Here's how the part is built. I have some questions about the finished solid (model axes, mm). A direction names the side the tool comes from. Coordinates: 2 decimals unless noted, no trailing zeros. Loops run counter-clockwise (first coordinate to the right, second up) from the corner with the lowest first, then second, coordinate; pieces in that order, holes last.
from build123d import *

# Parameters (mm, degrees)
F0_W     = 457.2
F0_H     = 342.9
F1_DEPTH = 12.7
F2_W     = 355.6
F2_H     = 241.3
F3_DEPTH = 25.4
F4_W     = 25.4
F4_H     = 127
F5_DEPTH = 25.4
F6_R     = 12.7


with BuildPart() as f1:
    # F0 (on Top) → F1 (new body)
    with BuildSketch(Plane.XY):
        with Locations((184.6840278864, 135.7329336226)):
            Rectangle(F0_W, F0_H)
    extrude(amount=F1_DEPTH)

    # F2 (on face) → F3 (cut)
    with BuildSketch(Plane.XY.offset(12.7)):
        with Locations((184.6840278864, 135.7329336226)):
            Rectangle(F2_W, F2_H)
    extrude(amount=-F3_DEPTH, mode=Mode.SUBTRACT)

    # F4 (on face) → F5 (cut)
    with BuildSketch(Plane.XY.offset(12.7)):
        with Locations((-5.8159721136, 135.7329336226)):
            Rectangle(F4_W, F4_H)
        with Locations((375.1840278864, 135.7329336226)):
            Rectangle(F4_W, F4_H)
    extrude(amount=-F5_DEPTH, mode=Mode.SUBTRACT)

    # F6
    f6_edges = [f1.edges().sort_by_distance(p)[0] for p in [
        (-18.515972, 199.232934, 6.35),
        (387.884028, 199.232934, 6.35),
        (-18.515972, 72.232934, 6.35),
        (387.884028, 72.232934, 6.35),
    ]]
    fillet(f6_edges, radius=F6_R)


solid = f1.part
Q1. Please list where these lines run through material, in increasing order: probe 1 along Y at (x, z) = (128, 1.5); probe 2 along X at (y, z) = (182, 9.25); probe 3 along Y at (x, z) = (-3.5, 7.75).
Q2. We'd pull the mould along X, two halves only. Please class faces 3 (the flat face through (181, -35.717, 6)), 4 (the flat face through (-43.916, 133, 6)), 5 (the flat face through (362.484, 43, 6)): pulls with the +X half, pulls with the -X half, needs draft (parallel to the pull), parting line crosses it, or undercut.
Q3. Will this pin go through, and if not, where does the flat tip stop? P1, Ø8, axis at x = 180.5, y = 251, coming from the -Z side.
Q4. Suppose I cut it at C-C on z = 2. Write out the boundary of the cut face in (x, y), and give its area (3 significant figures).
Q5. Suppose I cut it at B-B on x = 29. Write out the boundary of the cut face in (y, z), and give its area (3 significant figures).
Q6. For faces 1 (the flat face through (184, 264, 12.7)), 2 (the flat face through (362.484, 227, 6)), which set-ups out of +Z, -Z, +X, -X, +Y, -Y let a thin tool reach every point of the face, with its end or its side?
Q7. Suppose I cut it at A-A on y = 32. Write out the boundary of the cut face in (x, z), and give its area (3 significant figures).
Check values:
1. probe 1: y = -35.72 to 15.08, 256.38 to 307.18
1. probe 2: x = -43.92 to -18.52, 387.88 to 413.28
1. probe 3: y = -35.72 to 72.23, 199.23 to 307.18
2. face 3: needs draft
2. face 4: pulls with the -X half
2. face 5: undercut
3. P1: passes through
4. outline: (-43.92, -35.72) - (413.28, -35.72) - (413.28, 307.18) - (-43.92, 307.18) - close; hole (-18.52, 84.93) arc R12.7 ccw to (-5.82, 72.23) - (6.88, 72.23) - (6.88, 15.08) - (362.48, 15.08) - (362.48, 72.23) - (375.18, 72.23) arc R12.7 ccw to (387.88, 84.93) - (387.88, 186.53) arc R12.7 ccw to (375.18, 199.23) - (362.48, 199.23) - (362.48, 256.38) - (6.88, 256.38) - (6.88, 199.23) - (-5.82, 199.23) arc R12.7 ccw to (-18.52, 186.53) - close
4. area: 64,700 mm2
5. outline: (-35.72, 0) - (15.08, 0) - (15.08, 12.7) - (-35.72, 12.7) - close; (256.38, 0) - (307.18, 0) - (307.18, 12.7) - (256.38, 12.7) - close
5. area: 1,290 mm2
6. face 1: +Z, +X, -X, +Y, -Y
6. face 2: +Z, -Z
7. outline: (-43.92, 0) - (6.88, 0) - (6.88, 12.7) - (-43.92, 12.7) - close; (362.48, 0) - (413.28, 0) - (413.28, 12.7) - (362.48, 12.7) - close
7. area: 1,290 mm2
